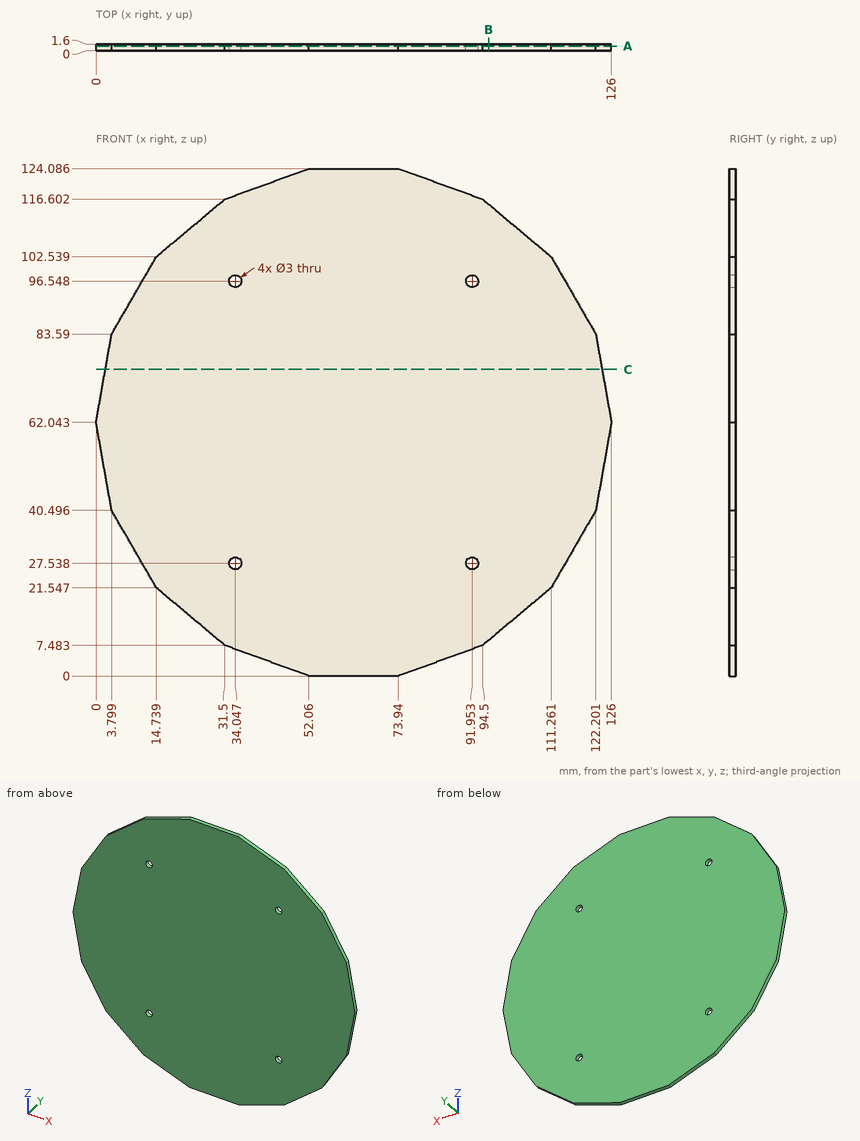
Design review of the part shown in the three views and the two pictorial views. Dimensions are in mm from the part's minimum x, y and z. Give positions to 0.01 mm unless a question says otherwise; leave off trailing zeros. Loops run counter-clockwise (first coordinate to the right, second up) from the corner with the lowest first, then second, coordinate; pieces in that order, holes last. Notation, with made-up numbers: (12, 62) -> (60, 62) arc R26 cw to (60, 85) -> close; hole circle Ø2 at (-26.5, -17). An arc over 180 degrees is marked (long way). One line per question, with ' | ' between items.
1) We need section A-A (y = 1.05). Write out the cut boundary in (x, z) (1 decimal).
Resolved:
outline: (0, 62) -> (3.8, 40.5) -> (14.7, 21.5) -> (31.5, 7.5) -> (52.1, 0) -> (73.9, 0) -> (94.5, 7.5) -> (111.3, 21.5) -> (122.2, 40.5) -> (126, 62) -> (122.2, 83.6) -> (111.3, 102.5) -> (94.5, 116.6) -> (73.9, 124.1) -> (52.1, 124.1) -> (31.5, 116.6) -> (14.7, 102.5) -> (3.8, 83.6) -> close; hole circle Ø3 at (34, 27.5); hole circle Ø3 at (34, 96.5); hole circle Ø3 at (92, 27.5); hole circle Ø3 at (92, 96.5)
2) We need section C-C (z = 75). Write out the cut boundary in (x, y) (1 decimal).
Resolved:
outline: (2.3, 0) -> (123.7, 0) -> (123.7, 1.6) -> (2.3, 1.6) -> close
3) Insertion check: pin 1 Ø5 at (x, z) = (34.05, 96.55) entering from -Y. The pin has a flat end and moves straight along its axis. Give the tip position at first contact, or say it passes through.
Resolved:
pin 1: stops at y = 0
4) We need section B-B (x = 96). Write out the cut boundary in (y, z).
Resolved:
outline: (0, 8.74) -> (1.6, 8.74) -> (1.6, 115.34) -> (0, 115.34) -> close
5) To check wall thickness, follow probe 1 along X at (y, z) = (1.15, 110); probe 2 along X at (y, z) = (1.2, 44.5); probe 3 along Z at (x, y) = (102, 1.1) (1 decimal). State the ranges of each line that lie inside material, in increasing order.
Resolved:
probe 1: x = 23.63 to 102.37 | probe 2: x = 3.09 to 122.91 | probe 3: z = 13.8 to 110.3
